from build123d import *

# Parameters (mm, degrees)
BOSS_EXTRUDE1_DEPTH = 28
SKETCH3_W           = 43
SKETCH3_H           = 5
BOSS_EXTRUDE2_DEPTH = 51
SKETCH4_R           = 8
CUT_EXTRUDE1_DEPTH  = 82.455509329
BOSS_EXTRUDE3_DEPTH = 12
BOSS_EXTRUDE4_DEPTH = 12
SKETCH5_R           = 2.25
CUT_EXTRUDE2_DEPTH  = 96.551033485
SKETCH8_W           = 55
SKETCH8_H           = 35
BOSS_EXTRUDE5_DEPTH = 6
CUT_EXTRUDE3_DEPTH  = 85.557672626
BOSS_EXTRUDE6_DEPTH = 4
SKETCH11_R          = 2.25
CUT_EXTRUDE4_DEPTH  = 81.783661714
CUT_EXTRUDE5_REACH  = 86.558
SKETCH12_R          = 2.25
CUT_EXTRUDE6_DEPTH  = 85.557672626
CUT_EXTRUDE7_DEPTH  = 92.793245939
SKETCH15_W          = 8
SKETCH15_H          = 28
CUT_EXTRUDE8_DEPTH  = 101.713703139


with BuildPart() as part:
    # Sketch2 → Boss-Extrude1 (new body)
    with BuildSketch(Plane(origin=(0, 0, 0), x_dir=(1, 0, 0), z_dir=(0, 1, 0))):
        Polygon((-16.5, 0), (0, 0), (0, 30), (10, 30), (10, -10), (-16.5, -10), align=None)
    extrude(amount=BOSS_EXTRUDE1_DEPTH)

    # Sketch3 → Boss-Extrude2 (add)
    with BuildSketch(Plane(origin=(0, 0, 0), x_dir=(1, 0, 0), z_dir=(0, 1, 0))):
        with Locations((31.5, -7.5)):
            Rectangle(SKETCH3_W, SKETCH3_H)
    extrude(amount=BOSS_EXTRUDE2_DEPTH)

    # Sketch4 → Cut-Extrude1 (cut, through all)
    with BuildSketch(Plane(origin=(0, 0, 5), x_dir=(-1, 0, 0), z_dir=(0, 0, -1))):
        with Locations((-32, 40)):
            Circle(SKETCH4_R)
    extrude(amount=-CUT_EXTRUDE1_DEPTH, mode=Mode.SUBTRACT)

    # Sketch6 → Boss-Extrude3 (add)
    with BuildSketch(Plane.ZY.offset(16.5)):
        with BuildLine():
            Line((10, 28), (10, 0))
            Line((10, 0), (18, 0))
            Line((18, 0), (18, 12))
            ThreePointArc((18, 12), (14, 16), (18, 20))
            Line((18, 20), (18, 28))
            Line((18, 28), (10, 28))
        make_face()
    extrude(amount=-BOSS_EXTRUDE3_DEPTH)

    # Sketch7 → Boss-Extrude4 (add)
    with BuildSketch(Plane(origin=(53, 0, 0), x_dir=(0, 0, -1), z_dir=(1, 0, 0))):
        with BuildLine():
            Line((-18, 12), (-18, 0))
            Line((-18, 0), (-5, 0))
            Line((-5, 0), (-5, 28))
            Line((-5, 28), (-18, 28))
            Line((-18, 28), (-18, 20))
            ThreePointArc((-18, 20), (-14, 16), (-18, 12))
        make_face()
    extrude(amount=BOSS_EXTRUDE4_DEPTH)

    # Sketch5 → Cut-Extrude2 (cut, through all)
    with BuildSketch(Plane.XY.offset(18)):
        with Locations((-10.5, 24)):
            Circle(SKETCH5_R)
        with Locations((-10.5, 8)):
            Circle(SKETCH5_R)
        with Locations((59, 8)):
            Circle(SKETCH5_R)
        with Locations((59, 24)):
            Circle(SKETCH5_R)
    extrude(amount=-CUT_EXTRUDE2_DEPTH, mode=Mode.SUBTRACT)

    # Sketch8 → Boss-Extrude5 (add)
    with BuildSketch(Plane(origin=(0, 0, 0), x_dir=(1, 0, 0), z_dir=(0, 1, 0))):
        with Locations((37.5, 12.5)):
            Rectangle(SKETCH8_W, SKETCH8_H)
    extrude(amount=BOSS_EXTRUDE5_DEPTH)

    # Sketch9 → Cut-Extrude3 (cut, through all)
    with BuildSketch(Plane(origin=(0, 6, 0), x_dir=(-1, 0, 0), z_dir=(0, 1, 0))):
        Polygon((-62.5, 5), (-55.5, 5), (-55.5, 0), (-56.75, 0), (-56.75, -5), (-61.25, -5), (-61.25, 0), (-62.5, 0), align=None)
    extrude(amount=-CUT_EXTRUDE3_DEPTH, mode=Mode.SUBTRACT)

    # Sketch10 → Boss-Extrude6 (add)
    with BuildSketch(Plane.ZY.offset(-10)):
        Polygon((-30, 0), (5, 51), (10, 51), (10, 36.428571429), (10, 0), (-15, 0), align=None)
    extrude(amount=BOSS_EXTRUDE6_DEPTH)

    # Sketch11 → Cut-Extrude4 (cut, through all)
    with BuildSketch(Plane(origin=(10, 0, 0), x_dir=(0, 0, -1), z_dir=(1, 0, 0))):
        with Locations((24, 10.5)):
            Circle(SKETCH11_R)
    extrude(amount=-CUT_EXTRUDE4_DEPTH, mode=Mode.SUBTRACT)

    # Sketch12 → Cut-Extrude5 (cut, up to next)
    with BuildSketch(Plane(origin=(0, 6, 0), x_dir=(-1, 0, 0), z_dir=(0, 1, 0)), mode=Mode.PRIVATE) as cut_extrude5_sk1:
        with Locations(Location((-18, -8, 0), (0, 0, 90))):
            Circle(SKETCH12_R)
    cut_extrude5_tool1 = extrude(cut_extrude5_sk1.sketch, amount=-CUT_EXTRUDE5_REACH, mode=Mode.PRIVATE) & part.part
    # Sketch12 → Cut-Extrude5 (cut, up to next)
    with BuildSketch(Plane(origin=(0, 6, 0), x_dir=(-1, 0, 0), z_dir=(0, 1, 0)), mode=Mode.PRIVATE) as cut_extrude5_sk2:
        with Locations(Location((-38, -8, 0), (0, 0, 90))):
            Circle(SKETCH12_R)
    cut_extrude5_tool2 = extrude(cut_extrude5_sk2.sketch, amount=-CUT_EXTRUDE5_REACH, mode=Mode.PRIVATE) & part.part
    add(cut_extrude5_tool1.solids().sort_by_distance((18, 6, -8))[0], mode=Mode.SUBTRACT)
    add(cut_extrude5_tool2.solids().sort_by_distance((38, 6, -8))[0], mode=Mode.SUBTRACT)

    # Sketch13 → Cut-Extrude6 (cut, through all)
    with BuildSketch(Plane(origin=(0, 6, 0), x_dir=(-1, 0, 0), z_dir=(0, 1, 0))):
        Polygon((-10, -30), (-65, -10), (-65, -30), align=None)
    extrude(amount=-CUT_EXTRUDE6_DEPTH, mode=Mode.SUBTRACT)

    # Sketch14 → Cut-Extrude7 (cut, through all)
    with BuildSketch(Plane.XY.offset(10)):
        with BuildLine():
            Line((41.204046185, 46.02374749), (53, 28))
            Line((53, 28), (53, 51))
            Line((53, 51), (32, 51))
            ThreePointArc((32, 51), (37.23157613, 49.67629119), (41.204046185, 46.02374749))
        make_face()
    extrude(amount=-CUT_EXTRUDE7_DEPTH, mode=Mode.SUBTRACT)

    # Sketch15 → Cut-Extrude8 (cut, through all)
    with BuildSketch(Plane.ZY.offset(16.5)):
        with Locations((14, 14)):
            Rectangle(SKETCH15_W, SKETCH15_H)
    extrude(amount=-CUT_EXTRUDE8_DEPTH, mode=Mode.SUBTRACT)


solid = part.part
Part model, mm, in its own coordinate system. A direction names the side the tool comes from. Give positions to 0.01 mm unless a question says otherwise; leave off trailing zeros. Write each loop counter-clockwise with the first axis right and the second up, starting at its lowest first coordinate (ties: lowest second). Pieces come first, ordered by that corner, then holes.
1) Pin check, flat tips, straight feed: pin 1 (5 mm diameter, centred on y = 10.5, z = -24, fed in from -X); pin 2 (1.5 mm diameter, centred on x = 58, z = 7.5, fed in from +Y); pin 3 (2.5 mm diameter, centred on x = 18, z = -8, fed in from +Y); pin 4 (5 mm diameter, centred on x = 38, z = -8, fed in from +Y). Stop position of each tip, or through.
Resolved:
pin 1: stops at x = 0
pin 2: stops at y = 28
pin 3: passes through
pin 4: stops at y = 6
2) Probe L1, parallel to Y at x = 59, z = 7.7; L2, parallel to Y at x = 32, z = 8; L3, parallel to Y at x = 4.75, z = -24. List the from-to ranges inside material, lowest first.
Resolved:
L1: y = 0 to 5.75, 10.25 to 21.75, 26.25 to 28
L2: y = 0 to 32, 48 to 51
L3: y = 0 to 8.25, 12.75 to 28
3) Cut at B-B on x = 59.5. Write the cut outline in (y, z), then the cut area to 3 significant figures.
Resolved:
outline: (0, -12) - (6, -12) - (6, -5) - (0, -5) - close; (0, 5) - (5.81, 5) - (5.81, 10) - (0, 10) - close; (10.19, 5) - (21.81, 5) - (21.81, 10) - (10.19, 10) - close; (26.19, 5) - (28, 5) - (28, 10) - (26.19, 10) - close
area: 138 mm2
4) Cut at D-D on z = -8. Write the cut outline in (x, y).
Resolved:
outline: (0, 0) - (15.75, 0) - (15.75, 6) - (10, 6) - (10, 32.06) - (6, 32.06) - (6, 28) - (0, 28) - close; (20.25, 0) - (35.75, 0) - (35.75, 6) - (20.25, 6) - close; (40.25, 0) - (65, 0) - (65, 6) - (40.25, 6) - close
5) Two-plate mould, pull along Y, no slides. Class faces 1 (the face through (5.07, 11.176, -26.146)), 2 (the face through (31, 6, -9)), 3 (the face through (37.9, 45.4, 7.5)), 4 (the face through (-8, 14, 0)): released by +Y, released by -Y, zero draft, split by the parting line, or undercut.
Resolved:
face 1: undercut
face 2: released by +Y
face 3: undercut
face 4: zero draft
6) Cut at A-A on y = 24. Write the cut outline in (x, z), then the cut area to 4 significant figures.
Resolved:
outline: (-16.5, 0) - (-12.75, 0) - (-12.75, 10) - (-16.5, 10) - close; (-8.25, 0) - (0, 0) - (0, -30) - (10, -30) - (10, 5) - (56.75, 5) - (56.75, 10) - (-8.25, 10) - close; (61.25, 5) - (65, 5) - (65, 10) - (61.25, 10) - close
area: 772.5 mm2
7) Cut at C-C on x = 28.5. Write the cut outline in (y, z).
Resolved:
outline: (0, -23.27) - (6, -23.27) - (6, 5) - (32.81, 5) - (32.81, 10) - (0, 10) - close; (47.19, 5) - (51, 5) - (51, 10) - (47.19, 10) - close
8) Which spindle directions (+Z, -Z, +X, -X, +Y, -Y) get a long thin tool onto all of the face, cutting with end or side? Do faces 5 (the face through (0, 14, -15)), 6 (the face through (6, 37, 2)), 7 (the face through (55.5, 3, 3)), 8 (the face through (59, 28, 7)). Say none if no direction does.
Resolved:
face 5: -Z, -X, +Y, -Y
face 6: +Z, -Z, -X, +Y
face 7: +Y, -Y
face 8: +Z, -Z, +X, +Y
